```python
from build123d import *

# Parameters (mm, degrees)
SKETCH_1_W      = 24
SKETCH_1_H      = 12
EXTRUDE_1_DEPTH = 16.3
SKETCH_2_W      = 24
SKETCH_2_H      = 12
SKETCH_2_W_2    = 8
SKETCH_2_H_2    = 8
SKETCH_2_W_3    = 4
SKETCH_2_R      = 1
EXTRUDE_3_DEPTH = 1.5
SKETCH_2_4_W    = 8
SKETCH_2_4_H    = 8
SKETCH_2_4_R    = 2.5
SKETCH_2_4_R_2  = 1.25
EXTRUDE_4_DEPTH = 10
SKETCH_2_5_R    = 2.5
SKETCH_2_5_R_2  = 1.25
EXTRUDE_5_DEPTH = 13.5
FILLET_1_R      = 1
FILLET_2_R      = 1
FILLET_3_R      = 1


with BuildPart() as part:
    # Sketch 1 → Extrude 1 (new body)
    with BuildSketch(Plane(origin=(0, 0, 0), x_dir=(1, 0, 0), z_dir=(0, 1, 0))):
        Rectangle(SKETCH_1_W, SKETCH_1_H)
    extrude(amount=EXTRUDE_1_DEPTH)

    # Sketch 2 → Extrude 3 (add)
    # profile 1 of 3: a face of its own
    with BuildSketch(Plane(origin=(0, 16.3, 0), x_dir=(1, 0, 0), z_dir=(0, 1, 0))):
        Rectangle(SKETCH_2_W, SKETCH_2_H)
        with Locations((6.23, 0)):
            Rectangle(SKETCH_2_W_2, SKETCH_2_H_2, mode=Mode.SUBTRACT)
    # profile 2 of 3: a face of its own
    with BuildSketch(Plane(origin=(0, 16.3, 0), x_dir=(1, 0, 0), z_dir=(0, 1, 0))):
        with Locations((-14, 0)):
            Rectangle(SKETCH_2_W_3, SKETCH_2_H)
        with Locations(Location((-14, 0, 0), (0, 0, 270))):
            Circle(SKETCH_2_R, mode=Mode.SUBTRACT)
    # profile 3 of 3: a face of its own
    with BuildSketch(Plane(origin=(0, 16.3, 0), x_dir=(1, 0, 0), z_dir=(0, 1, 0))):
        with Locations((14, 0)):
            Rectangle(SKETCH_2_W_3, SKETCH_2_H)
        with Locations(Location((14, 0, 0), (0, 0, 270))):
            Circle(SKETCH_2_R, mode=Mode.SUBTRACT)
    extrude(amount=EXTRUDE_3_DEPTH)

    # Sketch 2_4 → Extrude 4 (add)
    # profile 1 of 3: a face of its own
    with BuildSketch(Plane(origin=(0, 16.3, 0), x_dir=(1, 0, 0), z_dir=(0, 1, 0))):
        with Locations((6.23, 0)):
            Rectangle(SKETCH_2_4_W, SKETCH_2_4_H)
        with Locations((6.23, 0)):
            Circle(SKETCH_2_4_R, mode=Mode.SUBTRACT)
    # profile 2 of 3: a face of its own
    with BuildSketch(Plane(origin=(0, 16.3, 0), x_dir=(1, 0, 0), z_dir=(0, 1, 0))):
        with Locations((6.23, 0)):
            Circle(SKETCH_2_4_R)
        with Locations((6.23, 0)):
            Circle(SKETCH_2_4_R_2, mode=Mode.SUBTRACT)
    # profile 3 of 3: a face of its own
    with BuildSketch(Plane(origin=(0, 16.3, 0), x_dir=(1, 0, 0), z_dir=(0, 1, 0))):
        with Locations((6.23, 0)):
            Circle(SKETCH_2_4_R_2)
    extrude(amount=EXTRUDE_4_DEPTH)

    # Sketch 2_5 → Extrude 5 (add)
    with BuildSketch(Plane(origin=(0, 16.3, 0), x_dir=(1, 0, 0), z_dir=(0, 1, 0))):
        with Locations(Location((6.23, 0, 0), (0, 0, 270))):
            Circle(SKETCH_2_5_R)
        with Locations(Location((6.23, 0, 0), (0, 0, 270))):
            Circle(SKETCH_2_5_R_2, mode=Mode.SUBTRACT)
    extrude(amount=EXTRUDE_5_DEPTH)

    # Fillet 1
    fillet_1_edges = [part.edges().sort_by_distance(p)[0] for p in [
        (-16, 17.05, 6),
        (16, 17.05, 6),
        (16, 17.05, -6),
        (-16, 17.05, -6),
    ]]
    fillet(fillet_1_edges, radius=FILLET_1_R)

    # Fillet 2
    fillet_2_edges = [part.edges().sort_by_distance(p)[0] for p in [
        (10.23, 22.05, 4),
        (10.23, 22.05, -4),
        (2.23, 22.05, -4),
        (2.23, 22.05, 4),
    ]]
    fillet(fillet_2_edges, radius=FILLET_2_R)

    # Fillet 3
    fillet_3_edges = [part.edges().sort_by_distance(p)[0] for p in [
        (12, 8.15, 6),
        (-12, 8.15, 6),
        (-12, 8.15, -6),
        (12, 8.15, -6),
    ]]
    fillet(fillet_3_edges, radius=FILLET_3_R)


solid = part.part
```
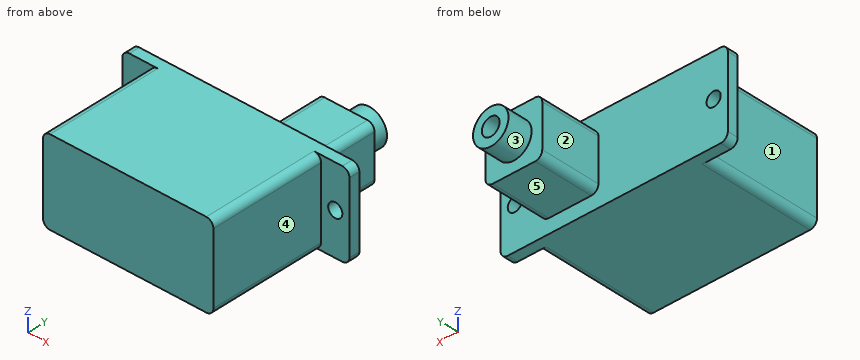
Geometry: final body of the model. Coordinates: model frame, mm. Face numbers are marked on the shaded views. A direction names the side the tool comes from. Round coordinates to 2 decimals unless told otherwise and drop trailing zeros. Loops run counter-clockwise (first coordinate to the right, second up) from the corner with the lowest first, then second, coordinate; pieces in that order, holes last. Notation, with made-up numbers: (-17.75, -4) -> (6.25, -4) arc R32 cw to (6.25, 29) -> close; hole circle Ø5 at (3.25, 89). An arc over 180 degrees is marked (long way). Write each question's results on one line, items separated by ' | '.
Item 1: Cut plane C-C on y = 21.5. Return the cut outline in (x, z), and give its area (3 significant figures).
Answers below:
outline: (2.23, -3) arc R1 ccw to (3.23, -4) -> (9.23, -4) arc R1 ccw to (10.23, -3) -> (10.23, 3) arc R1 ccw to (9.23, 4) -> (3.23, 4) arc R1 ccw to (2.23, 3) -> close | area: 63.1 mm²
Item 2: Cut plane B-B on z = 0. Return the cut outline in (x, y).
Answers below:
outline: (-16, 16.3) -> (-15, 16.3) -> (-15, 17.8) -> (-16, 17.8) -> close; (-13, 16.3) -> (-12, 16.3) -> (-12, 0) -> (12, 0) -> (12, 16.3) -> (13, 16.3) -> (13, 17.8) -> (10.23, 17.8) -> (10.23, 26.3) -> (8.73, 26.3) -> (8.73, 29.8) -> (7.48, 29.8) -> (7.48, 26.3) -> (4.98, 26.3) -> (4.98, 29.8) -> (3.73, 29.8) -> (3.73, 26.3) -> (2.23, 26.3) -> (2.23, 17.8) -> (-13, 17.8) -> close; (15, 16.3) -> (16, 16.3) -> (16, 17.8) -> (15, 17.8) -> close
Item 3: Line query: probe 1 along X at (y, z) = (16.85, 0); probe 2 along Y at (x, z) = (-5, -2); probe 3 along Y at (x, z) = (8, 2.25). Output: solid intervals per line, ascending. Write a range as [from, to].
Answers below:
probe 1: x = [-16, -15], [-13, 13], [15, 16] | probe 2: y = [0, 17.8] | probe 3: y = [0, 26.3]
Item 4: Cut plane A-A on x = 14. Return the cut outline in (y, z).
Answers below:
outline: (16.3, -6) -> (17.8, -6) -> (17.8, -1) -> (16.3, -1) -> close; (16.3, 1) -> (17.8, 1) -> (17.8, 6) -> (16.3, 6) -> close
Item 5: Cut plane D-D on x = 6.23. Return the cut outline in (y, z).
Answers below:
outline: (0, -6) -> (17.8, -6) -> (17.8, -4) -> (26.3, -4) -> (26.3, -2.5) -> (29.8, -2.5) -> (29.8, -1.25) -> (26.3, -1.25) -> (26.3, 1.25) -> (29.8, 1.25) -> (29.8, 2.5) -> (26.3, 2.5) -> (26.3, 4) -> (17.8, 4) -> (17.8, 6) -> (0, 6) -> close
Item 6: Pin query (flat end, axial travel): pin 1 Ø3 at (x, z) = (14, 0) entering from +Y; pin 2 Ø5 at (y, z) = (22.5, 1) entering from +X; pin 3 Ø1.8 at (y, z) = (20.5, -1) entering from -X. Return the tip coordinate at first contact, or that it passes through.
Answers below:
pin 1: stops at y = 17.8 | pin 2: stops at x = 10.23 | pin 3: stops at x = 2.23
Item 7: Set-up query: the marked faces 1, 2, 3, 4 and 5. Return all of +Z, -Z, +X, -X, +Y, -Y with unobstructed straight access to the full face (end or side cutting, diameter ignored); none if empty.
Answers below:
face 1: +Z, -Z, -X, -Y | face 2: +Z, -Z, -X, +Y | face 3: +Y | face 4: +Z, -Z, +X, -Y | face 5: -Z, +X, -X, +Y
